Part model, mm, in its own coordinate system. Face numbers are marked on the shaded views. A direction names the side the tool comes from. Give positions to 0.01 mm unless a question says otherwise; leave off trailing zeros. Order: outer loops, then holes, each group sorted by start corner. A loop starts at its lowest first (then second) coordinate and runs counter-clockwise, first axis right, second up. Notation, with made-up numbers: (77.25, -28.5) -> (120.25, -28.5) arc R23 ccw to (120.25, 6.5) -> close; hole circle Ø8 at (42, 22.25). An arc over 180 degrees is marked (long way). Write item = value, one per line. Start each with the question number.
Item 1: Band-saw the part on C-C on z = 3. Write the cut outline in (x, y).
Item 2: Band-saw the part on A-A on z = -1.5. Write the cut outline in (x, y).
Item 3: Pull direction Y, two halves, no side cores. Call the marked faces 1, 2 and 3: +Y half, -Y half, draft (parallel to the pull), parting line (faces both ways), or undercut.
Item 4: Band-saw the part on B-B on y = -11. Write the cut outline in (x, z), plus the area to 3 significant figures.
Item 5: Drill centre lines: line 1 along Z through (x, y) = (20.5, -7.5); line 2 along Y through (x, z) = (0, 2.25); line 3 along Y through (x, z) = (24.5, -9.5). Where is each one in solid material? Low to high.
Item 6: Tool access for the marked faces 4, 5, 6 and 7: list every direction of +Z, -Z, +X, -X, +Y, -Y with a clear straight run to the whole face (end or side of a thin tool).
Item 7: Flat gauge pins, fed straight in: P1, Ø3, axis at x = 22, z = -13.5, coming from the -Y side; P2, Ø6, axis at x = 17.5, z = -2, coming from the +Y side; P3, Ø2, axis at x = 7, z = 2, coming from the +Y side. Where does each tip first touch, or does it go through?
Item 8: Band-saw the part on D-D on x = 20.5. Write the cut outline in (y, z).
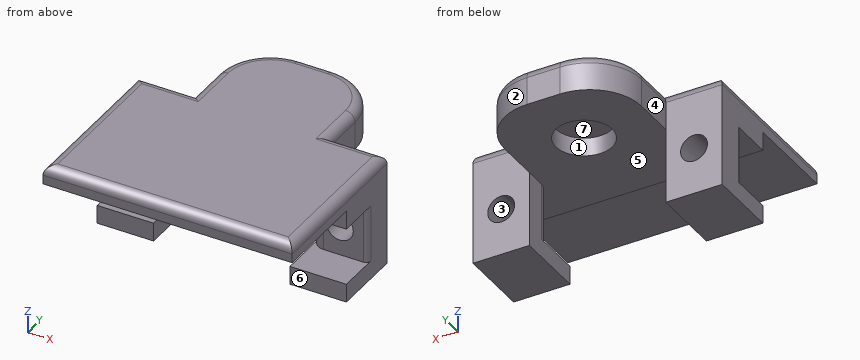
```python
from build123d import *

# Parameters (mm, degrees)
SKETCH_1_W           = 53
SKETCH_1_H           = 35
EXTRUDE_1_DEPTH      = 3.92
SKETCH_2_W           = 12
SKETCH_2_H           = 27
CUT_EXTRUDE_1_DEPTH  = 4
EXTRUDE_2_DEPTH      = 16.08
EXTRUDE_2_DEPTH_BACK = 3.92
SKETCH_3_W           = 12
SKETCH_3_H           = 7
SKETCH_4_W           = 12
SKETCH_4_H           = 3.92
EXTRUDE_3_DEPTH      = 8
SKETCH_5_R           = 2.86
CUT_EXTRUDE_2_DEPTH  = 37.889245045
SKETCH_6_R           = 6
CUT_EXTRUDE_3_DEPTH  = 4
EXTRUDE_4_DEPTH      = 4
SKETCH_8_W           = 53
SKETCH_8_H           = 3.92
EXTRUDE_5_DEPTH      = 20
FILLET_1_R           = 2.5
FILLET_2_R           = 11
FILLET_3_R           = 1
FILLET_4_R           = 2


with BuildPart() as part:
    # 스케치1 → 보스-돌출1 (new body)
    with BuildSketch(Plane.XY):
        Rectangle(SKETCH_1_W, SKETCH_1_H)
    extrude(amount=EXTRUDE_1_DEPTH)

    # 스케치2 → 컷-돌출1 (cut)
    with BuildSketch(Plane.XY.offset(3.92)):
        with Locations((-20.5, 4)):
            Rectangle(SKETCH_2_W, SKETCH_2_H)
        with Locations((20.5, 4)):
            Rectangle(SKETCH_2_W, SKETCH_2_H)
    extrude(amount=-CUT_EXTRUDE_1_DEPTH, mode=Mode.SUBTRACT)

    # 스케치3 → 보스-돌출2 (add, two sides: drawn at the far end of the back side and taken through both)
    with BuildSketch(Plane(origin=(0, 0, 0), x_dir=(-1, 0, 0), z_dir=(0, 0, -1)).offset(-EXTRUDE_2_DEPTH_BACK)):
        with Locations((-20.5, -6)):
            Rectangle(SKETCH_3_W, SKETCH_3_H)
        with Locations((20.5, -6)):
            Rectangle(SKETCH_3_W, SKETCH_3_H)
    extrude(amount=EXTRUDE_2_DEPTH + EXTRUDE_2_DEPTH_BACK)

    # 스케치4 → 보스-돌출3 (add)
    with BuildSketch(Plane.XZ.offset(9.5)):
        with Locations((-20.5, -14.12)):
            Rectangle(SKETCH_4_W, SKETCH_4_H)
        with Locations((20.5, -14.12)):
            Rectangle(SKETCH_4_W, SKETCH_4_H)
    extrude(amount=EXTRUDE_3_DEPTH)

    # 스케치5 → 컷-돌출2 (cut, through all)
    with BuildSketch(Plane(origin=(0, -2.5, 0), x_dir=(1, 0, 0), z_dir=(0, 1, 0))):
        with Locations(Location((-20.5, 6.08, 0), (0, 0, 180))):
            Circle(SKETCH_5_R)
        with Locations((20.5, 6.08)):
            Circle(SKETCH_5_R)
    extrude(amount=-CUT_EXTRUDE_2_DEPTH, mode=Mode.SUBTRACT)

    # 스케치6 → 컷-돌출3 (cut)
    with BuildSketch(Plane.XY.offset(3.92)):
        with Locations((0, 2.5)):
            Circle(SKETCH_6_R)
    extrude(amount=-CUT_EXTRUDE_3_DEPTH, mode=Mode.SUBTRACT)

    # 스케치7 → 보스-돌출4 (add)
    with BuildSketch(Plane.XY.offset(3.92)):
        Polygon((-14.5, -2.5), (-26.5, -2.5), (-26.5, -17.5), (26.5, -17.5), (26.5, -2.5), (14.5, -2.5), (14.5, 17.5), (-14.5, 17.5), align=None)
    extrude(amount=EXTRUDE_4_DEPTH)

    # 스케치8 → 보스-돌출5 (add)
    with BuildSketch(Plane.XZ.offset(17.5)):
        with Locations((0, 5.96)):
            Rectangle(SKETCH_8_W, SKETCH_8_H)
    extrude(amount=EXTRUDE_5_DEPTH)

    # 필렛1
    fillet_1_edges = [part.edges().sort_by_distance(p)[0] for p in [
        (14.5, -9.5, -6.08),
        (-14.5, -9.5, -6.08),
    ]]
    fillet(fillet_1_edges, radius=FILLET_1_R)

    # 필렛2
    fillet_2_edges = [part.edges().sort_by_distance(p)[0] for p in [
        (-14.5, 17.5, 3.96),
        (14.5, 17.5, 3.96),
    ]]
    fillet(fillet_2_edges, radius=FILLET_2_R)

    # 필렛3
    fillet_3_edges = [part.edges().sort_by_distance(p)[0] for p in [
        (26.5, -9.5, -6.08),
        (-26.5, -9.5, -6.08),
    ]]
    fillet(fillet_3_edges, radius=FILLET_3_R)

    # 필렛4
    fillet_4_edges = [part.edges().sort_by_distance(p)[0] for p in [
        (-20.5, -2.5, 7.92),
        (-26.5, -20, 7.92),
        (26.5, -20, 7.92),
        (20.5, -2.5, 7.92),
        (14.5, 2, 7.92),
        (0, -37.5, 7.92),
        (-14.5, 2, 7.92),
        (0, 17.5, 7.92),
        (-11.278174593, 14.278174593, 7.92),
        (11.278174593, 14.278174593, 7.92),
    ]]
    fillet(fillet_4_edges, radius=FILLET_4_R)


solid = part.part
```
Values found:
q1.outline = (-26.5, -17.5) -> (26.5, -17.5) -> (26.5, -2.5) -> (14.5, -2.5) -> (14.5, 6.5) arc R11 ccw to (3.5, 17.5) -> (-3.5, 17.5) arc R11 ccw to (-14.5, 6.5) -> (-14.5, -2.5) -> (-26.5, -2.5) -> close; hole circle Ø12 at (0, 2.5)
q2.outline = (-26.5, -8.5) arc R1 ccw to (-25.5, -9.5) -> (-17, -9.5) arc R2.5 ccw to (-14.5, -7) -> (-14.5, -2.5) -> (-26.5, -2.5) -> close; (14.5, -7) arc R2.5 ccw to (17, -9.5) -> (25.5, -9.5) arc R1 ccw to (26.5, -8.5) -> (26.5, -2.5) -> (14.5, -2.5) -> close
q3.face_1 = undercut
q3.face_2 = +Y half
q3.face_3 = draft
q4.outline = (-26.5, -16.08) -> (-14.5, -16.08) -> (-14.5, -12.16) -> (-26.5, -12.16) -> close; (-26.5, 0) -> (26.5, 0) -> (26.5, 5.92) arc R2 ccw to (24.5, 7.92) -> (-24.5, 7.92) arc R2 ccw to (-26.5, 5.92) -> close; (14.5, -16.08) -> (26.5, -16.08) -> (26.5, -12.16) -> (14.5, -12.16) -> close
q4.area = 512 mm^2
q5.line_1 = -16.08 to -8.94, -3.22 to 7.92
q5.line_2 = -17.5 to -3.5, 8.5 to 17.5
q5.line_3 = -9.5 to -2.5
q6.face_4 = +Z, -Z, -X, +Y
q6.face_5 = -Y
q6.face_6 = -Z, +X, -X, -Y
q6.face_7 = -Z
q7.P1 = -17.5
q7.P2 = -2.5
q7.P3 = 17.21
q8.outline = (-37.5, 4) -> (-17.5, 4) -> (-17.5, 0) -> (-9.5, 0) -> (-9.5, -3.22) -> (-2.5, -3.22) -> (-2.5, 5.92) arc R2 ccw to (-4.5, 7.92) -> (-35.5, 7.92) arc R2 ccw to (-37.5, 5.92) -> close; (-17.5, -16.08) -> (-2.5, -16.08) -> (-2.5, -8.94) -> (-9.5, -8.94) -> (-9.5, -12.16) -> (-17.5, -12.16) -> close
